```python
from build123d import *

# Parameters (mm, degrees)
SKETCH1_W           = 44.45
SKETCH1_H           = 44.45
SKETCH1_W_2         = 38.1
SKETCH1_H_2         = 38.1
BOSS_EXTRUDE1_DEPTH = 47.625


with BuildPart() as part:
    # Sketch1 → Boss-Extrude1 (new body, symmetric)
    with BuildSketch(Plane(origin=(0, 0, 0), x_dir=(0, 0, -1), z_dir=(1, 0, 0))):
        with Locations((22.225, 22.225)):
            Rectangle(SKETCH1_W, SKETCH1_H)
        with Locations((22.225, 22.225)):
            Rectangle(SKETCH1_W_2, SKETCH1_H_2, mode=Mode.SUBTRACT)
    extrude(amount=BOSS_EXTRUDE1_DEPTH, both=True)


solid = part.part
```
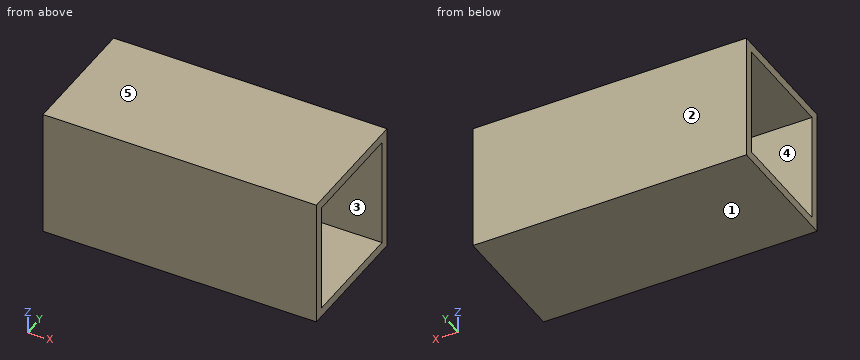
Build history of the part. All positions in model axes, mm. Face numbers are marked on the shaded views. A direction names the side the tool comes from. Round coordinates to 2 decimals unless told otherwise and drop trailing zeros. Order: outer loops, then holes, each group sorted by start corner. A loop starts at its lowest first (then second) coordinate and runs counter-clockwise, first axis right, second up. Notation, with made-up numbers: (19.25, 86) - (30.25, 86) arc R21 cw to (30.25, 97) - close; hole circle Ø10 at (56, 7). An arc over 180 degrees is marked (long way). Use a Markdown table: item, result.
1) Saw through at C-C on x = -10.5. Write the cut outline in (y, z) (3 decimals), and give its area (3 significant figures).
Recorded:
| item | result |
|---|---|
| outline | (0, -44.45) - (44.45, -44.45) - (44.45, 0) - (0, 0) - close; hole (3.175, -41.275) - (41.275, -41.275) - (41.275, -3.175) - (3.175, -3.175) - close |
| area | 524 mm² |
2) Saw through at A-A on z = -20. Write the cut outline in (x, y) (3 decimals), and give its area (3 significant figures).
Recorded:
| item | result |
|---|---|
| outline | (-47.625, 0) - (47.625, 0) - (47.625, 3.175) - (-47.625, 3.175) - close; (-47.625, 41.275) - (47.625, 41.275) - (47.625, 44.45) - (-47.625, 44.45) - close |
| area | 605 mm² |
3) Tool access for the marked faces 4 and 5: list every direction of +Z, -Z, +X, -X, +Y, -Y with a clear straight run to the whole face (end or side of a thin tool).
Recorded:
| item | result |
|---|---|
| face 4 | +X, -X |
| face 5 | +Z, +X, -X, +Y, -Y |
4) Saw through at B-B on y = 25. Write the cut outline in (x, z) (3 decimals), and give its area (3 significant figures).
Recorded:
| item | result |
|---|---|
| outline | (-47.625, -44.45) - (47.625, -44.45) - (47.625, -41.275) - (-47.625, -41.275) - close; (-47.625, -3.175) - (47.625, -3.175) - (47.625, 0) - (-47.625, 0) - close |
| area | 605 mm² |
5) Pull direction Z, two halves, no side cores. Call the marked faces 1, 2 and 3: pulls with the +Z half, pulls with the -Z half, needs draft (parallel to the pull), parting line crosses it, or undercut.
Recorded:
| item | result |
|---|---|
| face 1 | pulls with the -Z half |
| face 2 | needs draft |
| face 3 | undercut |
6) Wall check: L1, parallel to Z at x = -25, y = 12 (3 decimals); L2, parallel to Y at x = 27, z = -35.5 (3 decimals). Give the ranges that are in metal, low to high.
Recorded:
| item | result |
|---|---|
| L1 | z = -44.45 to -41.275, -3.175 to 0 |
| L2 | y = 0 to 3.175, 41.275 to 44.45 |
7) Flat gauge pin, fed straight in: pin 1 Ø10 at (y, z) = (31, -35) entering from +X. Where does the tip first touch, or does it go through?
Recorded:
| item | result |
|---|---|
| pin 1 | passes through |
